CAD build for the part. Positions are in the model's coordinates, mm. Coordinates: 2 decimals unless noted, no trailing zeros. Write each loop counter-clockwise with the first axis right and the second up, starting at its lowest first coordinate (ties: lowest second). Pieces come first, ordered by that corner, then holes. Notation, with made-up numbers: M -19.75,83.25 L -2.75,83.25 A17 ccw -2.75,109.25 Z; hole C 1.25,22.5 d10. An arc over 180 degrees is marked long. Put each result on its own line as item: value. Start each with the question number.
```python
from build123d import *

# Parameters (mm, degrees)
BOSS_EXTRUDE1_DEPTH = 4


with BuildPart() as part:
    # Sketch1 → Boss-Extrude1 (new body)
    with BuildSketch(Plane(origin=(0, 0, 0), x_dir=(1, 0, 0), z_dir=(0, 1, 0))):
        with BuildLine():
            Line((285.295698998, -100.459464193), (285.295698998, -116.089464193))
            ThreePointArc((285.295698998, -116.089464193), (269.186571963, -154.980337158), (230.295698998, -171.089464193))
            Line((230.295698998, -171.089464193), (5.265698998, -171.089464193))
            ThreePointArc((5.265698998, -171.089464193), (-33.625173967, -154.980337158), (-49.734301002, -116.089464193))
            Line((-49.734301002, -116.089464193), (-49.734301002, -26.829464193))
            ThreePointArc((-49.734301002, -26.829464193), (-33.625173967, 12.061408773), (5.265698998, 28.170535807))
            Line((5.265698998, 28.170535807), (230.295698998, 28.170535807))
            ThreePointArc((230.295698998, 28.170535807), (269.186571963, 12.061408773), (285.295698998, -26.829464193))
            Line((285.295698998, -26.829464193), (285.295698998, -42.459464193))
            Line((285.295698998, -42.459464193), (198.295698998, -42.459464193))
            Line((198.295698998, -42.459464193), (198.295698998, -95.459464193))
            ThreePointArc((198.295698998, -95.459464193), (195.36676681, -102.530532004), (188.295698998, -105.459464193))
            Line((188.295698998, -105.459464193), (173.295698998, -105.459464193))
            Line((173.295698998, -105.459464193), (173.295698998, -17.459464193))
            Line((173.295698998, -17.459464193), (258.794876179, -17.459464193))
            ThreePointArc((258.794876179, -17.459464193), (247.886889975, -2.528229656), (230.295698998, 3.170535807))
            Line((230.295698998, 3.170535807), (5.265698998, 3.170535807))
            ThreePointArc((5.265698998, 3.170535807), (-15.947504438, -5.616260757), (-24.734301002, -26.829464193))
            Line((-24.734301002, -26.829464193), (-24.734301002, -116.089464193))
            ThreePointArc((-24.734301002, -116.089464193), (-15.947504438, -137.302667628), (5.265698998, -146.089464193))
            Line((5.265698998, -146.089464193), (230.295698998, -146.089464193))
            ThreePointArc((230.295698998, -146.089464193), (247.886889975, -140.390698729), (258.794876179, -125.459464193))
            Line((258.794876179, -125.459464193), (258.794876179, -117.089464193))
            ThreePointArc((258.794876179, -117.089464193), (259.673555836, -114.968143849), (261.794876179, -114.089464193))
            Line((261.794876179, -114.089464193), (264.045287589, -114.089464193))
            ThreePointArc((264.045287589, -114.089464193), (271.1163554, -111.160532004), (274.045287589, -104.089464193))
            Line((274.045287589, -104.089464193), (274.045287589, -100.459464193))
            Line((274.045287589, -100.459464193), (285.295698998, -100.459464193))
        make_face()
    extrude(amount=BOSS_EXTRUDE1_DEPTH)


solid = part.part
```
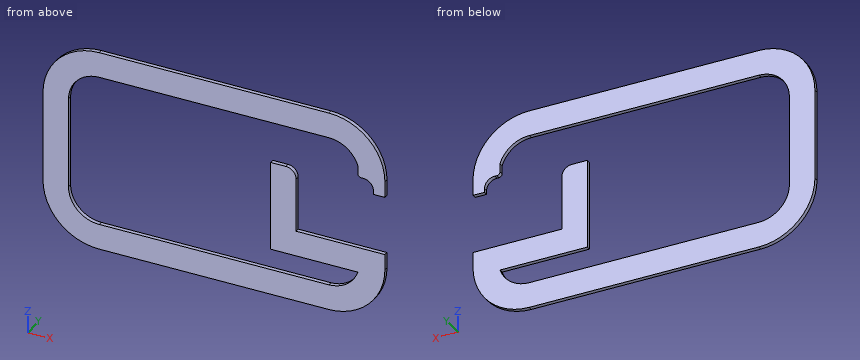
(1) Slice it at B-B, the plane z = 73. Write the cut outline in (x, y), then the cut area to 3 significant figures.
(2) Drop flat-ended pins along their axis: pin 1 (1.5 mm diameter, centred on y = 1.5, z = 135, fed in from +X); pin 2 (2 mm diameter, centred on y = 1, z = 50, fed in from +X); pin 3 (2 mm diameter, centred on y = 3, z = 123, fed in from -X). Give the stop position or say it passes through.
(3) Slice it at D-D, the plane x = 220. Write the cut outline in (y, z), then the cut area to 3 significant figures.
(4) Slice it at A-A, the plane x = 9. Write the cut outline in (y, z), then the cut area to 3 significant figures.
(5) Drill centre lines: line 1 (Z direction, x = 209, y = 1.8); line 2 (X direction, y = 0.2, z = 60); line 3 (Z direction, x = 116, y = 0.5). Where is each one in solid material? Low to high. Write a range as [from, to].
(6) Slice it at C-C, the plane y = 3.15. Write the cut outline in (x, z).
Result set:
1. outline: M -49.73,0 L -24.73,0 L -24.73,4 L -49.73,4 Z; M 173.3,0 L 198.3,0 L 198.3,4 L 173.3,4 Z
1. area: 200 mm^2
2. pin 1: stops at x = 282.21
2. pin 2: stops at x = 198.3
2. pin 3: stops at x = -49.42
3. outline: M 0,-28.17 L 4,-28.17 L 4,-3.17 L 0,-3.17 Z; M 0,17.46 L 4,17.46 L 4,42.46 L 0,42.46 Z; M 0,146.09 L 4,146.09 L 4,171.09 L 0,171.09 Z
3. area: 300 mm^2
4. outline: M 0,-28.17 L 4,-28.17 L 4,-3.17 L 0,-3.17 Z; M 0,146.09 L 4,146.09 L 4,171.09 L 0,171.09 Z
4. area: 200 mm^2
5. line 1: z = [-28.17, -3.17], [17.46, 42.46], [146.09, 171.09]
5. line 2: x = [-49.73, -24.73], [173.3, 198.3]
5. line 3: z = [-28.17, -3.17], [146.09, 171.09]
6. outline: M -49.73,26.83 A55 ccw 5.27,-28.17 L 230.3,-28.17 A55 ccw 285.3,26.83 L 285.3,42.46 L 198.3,42.46 L 198.3,95.46 A10 ccw 188.3,105.46 L 173.3,105.46 L 173.3,17.46 L 258.79,17.46 A30 cw 230.3,-3.17 L 5.27,-3.17 A30 cw -24.73,26.83 L -24.73,116.09 A30 cw 5.27,146.09 L 230.3,146.09 A30 cw 258.79,125.46 L 258.79,117.09 A3 ccw 261.79,114.09 L 264.05,114.09 A10 cw 274.05,104.09 L 274.05,100.46 L 285.3,100.46 L 285.3,116.09 A55 ccw 230.3,171.09 L 5.27,171.09 A55 ccw -49.73,116.09 Z
